Design review of the part built by this model. Coordinates are the model's own, in mm. A direction names the side the tool comes from. Round coordinates to 2 decimals unless told otherwise and drop trailing zeros. Loops run counter-clockwise (first coordinate to the right, second up) from the corner with the lowest first, then second, coordinate; pieces in that order, holes last. Notation, with made-up numbers: M -10,-18.75 L 29,-18.75 A17 cw 29,-4.75 Z; hole C -25,64 d10. An arc over 180 degrees is marked long. Use a Markdown table: item, result.
from build123d import *

# Parameters (mm, degrees)
SKETCH1_R             = 1.25
BOSS_EXTRUDE1_DEPTH   = 8
CUT_EXTRUDE2_DEPTH    = 61.942595941
M3X0_5_TAPPED_HOLE1_D = 2.5
SKETCH7_W             = 8
SKETCH7_H             = 0.5
CUT_EXTRUDE3_DEPTH    = 61.942595941
SKETCH8_R             = 2
CUT_EXTRUDE4_DEPTH    = 57.231663678
SKETCH9_W             = 38.671878994
SKETCH9_H             = 56.45112265
CUT_EXTRUDE5_DEPTH    = 8.1
CUT_EXTRUDE6_DEPTH    = 3
CUT_EXTRUDE8_START    = -1
CUT_EXTRUDE8_DEPTH    = 1


with BuildPart() as part:
    # Sketch1 → Boss-Extrude1 (new body)
    with BuildSketch(Plane(origin=(0, 0, 0), x_dir=(0, 0, -1), z_dir=(1, 0, 0))):
        with BuildLine():
            Line((0, 0), (0, 16))
            Line((0, 16), (-23.49505807, 51.650837947))
            ThreePointArc((-23.49505807, 51.650837947), (-27.398738146, 52.653965259), (-28.777698581, 48.866690426))
            Line((-28.777698581, 48.866690426), (-17, 20))
            Line((-17, 20), (-17, 0))
            Line((-17, 0), (0, 0))
        make_face()
        with Locations((-26, 50)):
            Circle(SKETCH1_R, mode=Mode.SUBTRACT)
    boss_extrude1 = extrude(amount=BOSS_EXTRUDE1_DEPTH)

    # Sketch3 → Cut-Extrude2 (cut, through all)
    with BuildSketch(Plane(origin=(0, 0, 0), x_dir=(-1, 0, 0), z_dir=(0, 0, -1))):
        Polygon((-8, 0), (-5, 0), (-3, 4), (-8, 4), align=None)
    cut_extrude2 = extrude(amount=-CUT_EXTRUDE2_DEPTH, mode=Mode.SUBTRACT)

    # M3x0.5 Tapped Hole1 (through all)
    with Locations(Plane(origin=(8, 7, 3), x_dir=(0, 0, 1), z_dir=(1, 0, 0))):
        with Locations((0, 0)):
            m3x0_5_tapped_hole1 = Hole(M3X0_5_TAPPED_HOLE1_D / 2)

    # Sketch7 → Cut-Extrude3 (cut, through all)
    with BuildSketch(Plane(origin=(0, 0, 0), x_dir=(-1, 0, 0), z_dir=(0, 0, -1))):
        with Locations((-4, 0.25)):
            Rectangle(SKETCH7_W, SKETCH7_H)
    cut_extrude3 = extrude(amount=-CUT_EXTRUDE3_DEPTH, mode=Mode.SUBTRACT)

    # Sketch8 → Cut-Extrude4 (cut, through all)
    with BuildSketch(Plane.XY.offset(17)):
        with Locations((4, 12)):
            Circle(SKETCH8_R)
    cut_extrude4 = extrude(amount=-CUT_EXTRUDE4_DEPTH, mode=Mode.SUBTRACT)

    # Mirror1: Boss-Extrude1, Cut-Extrude2, M3x0.5 Tapped Hole1, Cut-Extrude3, Cut-Extrude4 across plane
    add(boss_extrude1.mirror(Plane(origin=(0, 50, 26), x_dir=(0, 0, 1), z_dir=(1, 0, 0))))
    add(cut_extrude2.mirror(Plane(origin=(0, 50, 26), x_dir=(0, 0, 1), z_dir=(1, 0, 0))), mode=Mode.SUBTRACT)
    add(m3x0_5_tapped_hole1.mirror(Plane(origin=(0, 50, 26), x_dir=(0, 0, 1), z_dir=(1, 0, 0))), mode=Mode.SUBTRACT)
    add(cut_extrude3.mirror(Plane(origin=(0, 50, 26), x_dir=(0, 0, 1), z_dir=(1, 0, 0))), mode=Mode.SUBTRACT)
    add(cut_extrude4.mirror(Plane(origin=(0, 50, 26), x_dir=(0, 0, 1), z_dir=(1, 0, 0))), mode=Mode.SUBTRACT)

    # Sketch9 → Cut-Extrude5 (cut)
    with BuildSketch(Plane(origin=(8, 0, 0), x_dir=(0, 0, -1), z_dir=(1, 0, 0))):
        with Locations((-19.335939497, 28.725561325)):
            Rectangle(SKETCH9_W, SKETCH9_H)
    extrude(amount=-CUT_EXTRUDE5_DEPTH, mode=Mode.SUBTRACT)

    # Sketch10 → Cut-Extrude6 (cut)
    with BuildSketch(Plane(origin=(0, 0, 0), x_dir=(-1, 0, 0), z_dir=(0, 0, -1))):
        Polygon((4.75, 0.5), (3, 4), (0.1, 4), (0.1, 0.5), align=None)
    extrude(amount=-CUT_EXTRUDE6_DEPTH, mode=Mode.SUBTRACT)

    # Sketch12 → Cut-Extrude8 (cut)
    with BuildSketch(Plane(origin=(-0.1, 0, 0), x_dir=(0, 0, -1), z_dir=(1, 0, 0)).offset(CUT_EXTRUDE8_START)):
        with BuildLine():
            Line((-17, 20), (-28.777698581, 48.866690426))
            ThreePointArc((-28.777698581, 48.866690426), (-27.398738146, 52.653965259), (-23.49505807, 51.650837947))
            Line((-23.49505807, 51.650837947), (0, 16))
            Line((0, 16), (-17, 20))
        make_face()
    extrude(amount=CUT_EXTRUDE8_DEPTH, mode=Mode.SUBTRACT)


solid = part.part
1. Insertion check: pin 1 (3 mm diameter, centred on y = 22.5, z = 19, fed in from -X); pin 2 (3 mm diameter, centred on x = -1.5, z = 16.5, fed in from +Y); pin 3 (12 mm diameter, centred on y = 29.5, z = 25, fed in from +X); pin 4 (2 mm diameter, centred on x = -5.5, z = 24, fed in from -Y). Each pin has a flat end and moves straight along its axis. Give the tip position at first contact, or say it passes through.
Check values:
| item | result |
|---|---|
| pin 1 | stops at x = -8 |
| pin 2 | stops at y = 43.31 |
| pin 3 | stops at x = -1.1 |
| pin 4 | stops at y = 34.71 |
2. Take a section at D-D on z = 13.5. Give the boundary of the cut face in (x, y).
Check values:
| item | result |
|---|---|
| outline | M -8,4 L -3,4 L -4.75,0.5 L -0.1,0.5 L -0.1,19.18 L -1.1,19.18 L -1.1,36.48 L -8,36.48 Z; hole C -4,12 d4 |
3. Wall thickness on line 1 along Z through (x, y) = (-2.5, 7); line 2 along Y through (x, z) = (-5.75, 3); line 3 along Y through (x, z) = (-3.5, 4.75): over which ranges is each line inside the solid? List them lowest first. Write a range as from..to.
Check values:
| item | result |
|---|---|
| line 1 | z = 0..1.75, 4.25..17 |
| line 2 | y = 4..5.75, 8.25..11.03, 12.97..20.55 |
| line 3 | y = 0.5..3, 4..10.06, 13.94..23.21 |
4. Take a section at A-A on x = -4. Give the boundary of the cut face in (y, z).
Check values:
| item | result |
|---|---|
| outline | M 0.5,3 L 2,3 L 2,17 L 0.5,17 Z; M 4,0 L 10,0 L 10,17 L 4,17 Z; M 14,0 L 16,0 L 51.65,23.5 A3 ccw 48.87,28.78 L 20,17 L 14,17 Z; hole C 7,3 d2.5; hole C 50,26 d2.5 |
5. Machinability: for faces 1 (the face through (-2, 2, 3)), 2 (the face through (-8, 23, 15)), 3 (the face through (-4, 2, 10)), 4 (the face through (-2, 10, 17)), which of the approach directions +Z, -Z, +X, -X, +Y, -Y give a long, thin tool a straight path to every point of the face, cutting with its end or side? Answer none if there is none.
Check values:
| item | result |
|---|---|
| face 1 | -Z, +X, -X, -Y |
| face 2 | +Z, -Z, -X, +Y, -Y |
| face 3 | +Z, -Z, -X |
| face 4 | +Z, +X, -X, -Y |
6. Take a section at C-C on z = 26. Give the boundary of the cut face in (x, y).
Check values:
| item | result |
|---|---|
| outline | M -8,42.06 L -1.1,42.06 L -1.1,48.75 L -8,48.75 Z; M -8,51.25 L -1.1,51.25 L -1.1,53 L -8,53 Z |
7. Take a section at B-B on y = 7. Give the boundary of the cut face in (x, z).
Check values:
| item | result |
|---|---|
| outline | M -8,0 L -0.1,0 L -0.1,1.75 L -8,1.75 Z; M -8,4.25 L -0.1,4.25 L -0.1,17 L -8,17 Z |
8. The part is to be moulded in two halves that separate along X. For faces 5 (the face through (-1.1, 32, 17)), 6 (the face through (-4, 14, 9)), 7 (the face through (-0.61, 17.97, 8.38)), say which applies: pulls with the +X half, pulls with the -X half, needs draft (parallel to the pull), parting line crosses it, or undercut.
Check values:
| item | result |
|---|---|
| face 5 | pulls with the +X half |
| face 6 | undercut |
| face 7 | needs draft |
